Read the model definition and answer for the solid it produces. Units are mm, in the model's axes. A direction names the side the tool comes from. Round coordinates to 2 decimals unless told otherwise and drop trailing zeros. Write each loop counter-clockwise with the first axis right and the second up, starting at its lowest first coordinate (ties: lowest second). Pieces come first, ordered by that corner, then holes. Notation, with made-up numbers: (-9.75, 63) - (33.25, 63) arc R20 cw to (33.25, 84) - close; hole circle Ø8 at (-37, 86). An arc over 180 degrees is marked (long way). Use one line per item in the form item = value. Start each with the question number.
1) Each of these flat-tipped pins is pushed along its axis until it touches: pin 1 (7.5 mm diameter, centred on y = 4.5, z = 13, fed in from -X); pin 2 (1.5 mm diameter, centred on x = 15, z = 9.5, fed in from +Y); pin 3 (8 mm diameter, centred on y = 47, z = 8.5, fed in from -X). Where does it stop, or does it pass through?
2) For faces 1 (the face through (137, -5, 31)), 2 (the face through (100.325, 34.51, -38.605)), 3 (the face through (24.583, 1.487, -38.395)), 4 (the face through (159.7, 8.38, 38.39)), determine the directions among +Z, -Z, +X, -X, +Y, -Y from which every point of the face is accessible in a straight line to the end or side of a thin tool.
3) The part is cut by section C-C, the plane z = -26.5. Give the vertices of the cut face in (x, y).
4) The part is cut by section D-D, the plane y = 64.5. Give the vertices of the cut face in (x, z).
5) The part is cut by section A-A, the plane x = 138. Give the vertices of the cut face in (y, z).
6) Consider line 1 along Z through (x, y) = (74, 74); line 2 along X through (y, z) = (68, 0); line 3 along X through (y, z) = (9, 36.5). Determine where each line is inside the solid, lowest interval first. Write a range as from..to.
7) For a pull along Z with two mould halves and no side action, classify faces 5 (the face through (90, 0, 1)), 6 (the face through (73, 22, 46)), 7 (the face through (146, 70, 0)) as released by +Z, released by -Z, zero draft, split by the parting line, or undercut.
8) The part is cut by section B-B, the plane y = 12. Give the vertices of the cut face in (x, z).
from build123d import *

# Parameters (mm, degrees)
EXTRUDE1_DEPTH      = 70
EXTRUDE2_DEPTH      = 70
EXTRUDE2_DEPTH_BACK = 90
SKETCH3_R           = 31
EXTRUDE3_DEPTH      = 86
EXTRUDE4_REACH      = 88
SKETCH4_R           = 15
SKETCH5_R           = 15
SKETCH5_R_2         = 22
EXTRUDE5_DEPTH      = 15


with BuildPart() as part:
    # Sketch1 → Extrude1 (new body)
    with BuildSketch(Plane(origin=(0, 0, 0), x_dir=(1, 0, 0), z_dir=(0, 1, 0))):
        Polygon((178, 31), (178, -31), (113, -31), (88, -46), (58, -46), (43, -31), (0, -31), (0, 31), (43, 31), (58, 46), (88, 46), (113, 31), align=None)
    extrude(amount=EXTRUDE1_DEPTH)

    # Sketch2 → Extrude2 (cut, two sides)
    with BuildSketch(Plane.XY.offset(31)) as extrude2_sk:
        Polygon((113, 70), (0, 70), (0, 15), align=None)
    extrude(amount=EXTRUDE2_DEPTH, mode=Mode.SUBTRACT)
    extrude(extrude2_sk.sketch, amount=-EXTRUDE2_DEPTH_BACK, mode=Mode.SUBTRACT)

    # Sketch3 → Extrude3 (add)
    with BuildSketch(Plane(origin=(0, 0, 0), x_dir=(1, 0, 0), z_dir=(0, 1, 0))):
        with Locations(Location((74, 0, 0), (0, 0, 180))):  # turned: the seam where the file's is
            Circle(SKETCH3_R)
    extrude(amount=EXTRUDE3_DEPTH)

    # Extrude4: up to this plane
    extrude4_end = Plane(origin=(113, 70, 101), z_dir=(-0.43763961, 0.899150472, 0))
    # Sketch4 → Extrude4 (cut, up to the surface)
    with BuildSketch(Plane(origin=(0, 86, 0), x_dir=(1, 0, 0), z_dir=(0, 1, 0)), mode=Mode.PRIVATE) as extrude4_sk1:
        with Locations(Location((74, 0, 0), (0, 0, 270))):  # turned: the seam where the file's is
            Circle(SKETCH4_R)
    extrude4_tool1 = split(extrude(extrude4_sk1.sketch, amount=-EXTRUDE4_REACH, mode=Mode.PRIVATE), bisect_by=extrude4_end, keep=Keep.BOTH, mode=Mode.PRIVATE)
    add(extrude4_tool1.solids().sort_by_distance((74, 86, 0))[0], mode=Mode.SUBTRACT)

    # Sketch5 → Extrude5 (add)
    with BuildSketch(Plane.XY.offset(31)):
        with Locations(Location((10, 5, 0), (0, 0, 88.976968381))):  # turned: the seam where the file's is
            Circle(SKETCH5_R)
        with Locations(Location((138, 12, 0), (0, 0, 213.055731151))):  # turned: the seam where the file's is
            Circle(SKETCH5_R_2)
    extrude5 = extrude(amount=EXTRUDE5_DEPTH)

    # Mirror1: Extrude5 across plane
    add(extrude5.mirror(Plane.XY))


solid = part.part
Geometry results:
q1.pin_1 = 0
q1.pin_2 = 22.67
q1.pin_3 = 43.33
q2.face_1 = +X, -X, -Y
q2.face_2 = -Z, +Y, -Y
q2.face_3 = -Z
q2.face_4 = +Z
q3.outline = (0, 0) - (178, 0) - (178, 70) - (113, 70) - (90.09, 58.85) - (90.09, 86) - (57.91, 86) - (57.91, 43.19) - (0, 15) - close
q4.outline = (101.7, -37.78) - (113, -31) - (178, -31) - (178, 31) - (113, 31) - (101.7, 37.78) - (101.7, 13.92) arc R31 ccw (long way) to (101.7, -13.92) - close; hole circle Ø30 at (74, 0)
q5.outline = (-10, -46) - (34, -46) - (34, -31) - (70, -31) - (70, 31) - (34, 31) - (34, 46) - (-10, 46) - (-10, 31) - (0, 31) - (0, -31) - (-10, -31) - close
q6.line_1 = -31..-15, 15..31
q6.line_2 = 43..59, 89..105, 108.89..178
q6.line_3 = -4.46..24.46, 48.5..103.83, 116.21..159.79
q7.face_5 = undercut
q7.face_6 = released by +Z
q7.face_7 = zero draft
q8.outline = (-3.27, -46) - (23.27, -46) - (23.27, -31) - (43, -31) - (58, -46) - (88, -46) - (113, -31) - (116, -31) - (116, -46) - (160, -46) - (160, -31) - (178, -31) - (178, 31) - (160, 31) - (160, 46) - (116, 46) - (116, 31) - (113, 31) - (88, 46) - (58, 46) - (43, 31) - (23.27, 31) - (23.27, 46) - (-3.27, 46) - (-3.27, 31) - (0, 31) - (0, -31) - (-3.27, -31) - close
